For this review, use the dimensioned drawing (mm, ordinates from the lowest corner) and the shaded views. Give positions to 0.01 mm unless a question says otherwise; leave off trailing zeros. Write each loop counter-clockwise with the first axis right and the second up, starting at its lowest first coordinate (ties: lowest second). Pieces come first, ordered by that corner, then holes.
1) We need section D-D on x = 36. Give the boundary of the cut face in (y, z).
2) Draft analysis for pull direction Z (two halves, no side actions). For the marked faces 1 and 2, state which applies: pulls with the +Z half, pulls with the -Z half, needs draft (parallel to the pull), parting line crosses it, or undercut.
3) We need section B-B on x = 320. Give the boundary of the cut face in (y, z), and give its area (3 significant figures).
4) For P1, Ø11, axis at x = 307, z = 14.5, coming from the +Y side; P2, Ø6, axis at x = 317.5, y = 441.5, coming from the +Z side; P3, Ø11, axis at y = 101, z = 17, coming from the -X side; P4, Ø8, axis at x = 318, z = 14.5, coming from the -Y side, all flat-tipped, find the tip position at first contact; note any pin that passes through.
5) Wall thickness on line 1 along Y through (x, z) = (336, 12); line 2 along Z through (x, y) = (162, 141.5); line 3 along X through (y, z) = (475, 13.75): over which ranges is each line inside the solid? List them lowest first.
6) We need section C-C on y = 266. Give the boundary of the cut face in (x, z), and give its area (3 significant figures).
7) We need section A-A on z = 16.5. Give the boundary of the cut face in (x, y).
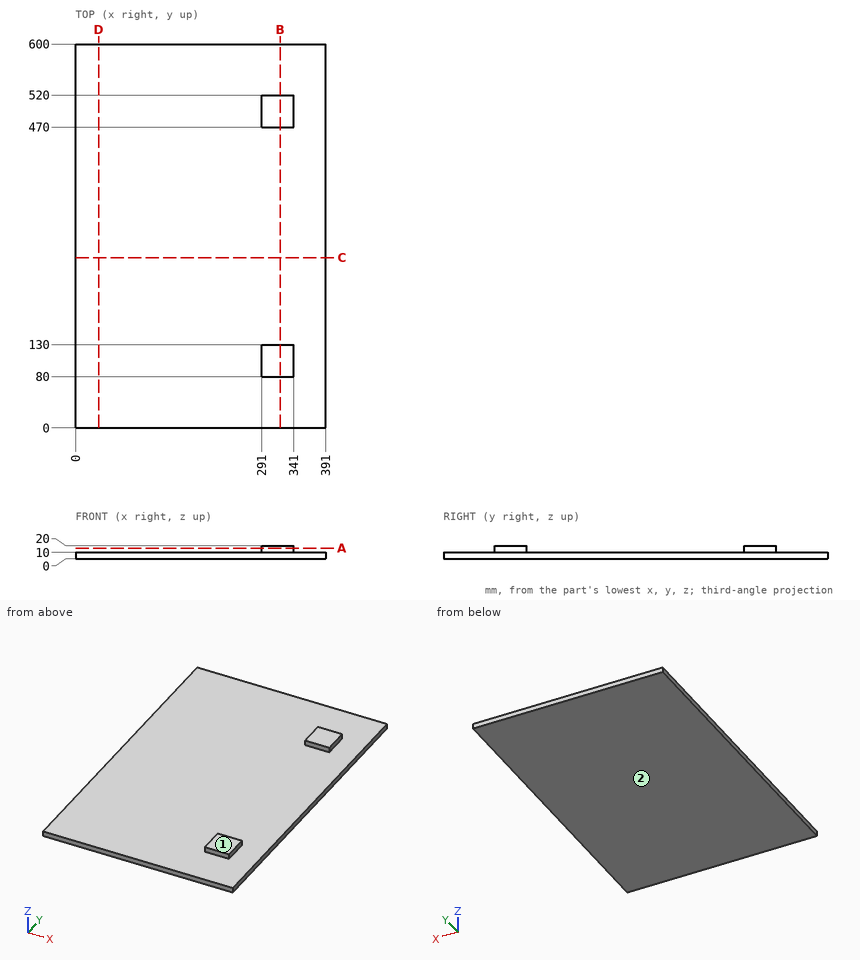
Results list:
1. outline: (0, 0) - (600, 0) - (600, 10) - (0, 10) - close
2. face 1: pulls with the +Z half
2. face 2: pulls with the -Z half
3. outline: (0, 0) - (600, 0) - (600, 10) - (520, 10) - (520, 20) - (470, 20) - (470, 10) - (130, 10) - (130, 20) - (80, 20) - (80, 10) - (0, 10) - close
3. area: 7,000 mm2
4. P1: stops at y = 600
4. P2: stops at z = 10
4. P3: stops at x = 291
4. P4: stops at y = 80
5. line 1: y = 80 to 130, 470 to 520
5. line 2: z = 0 to 10
5. line 3: x = 291 to 341
6. outline: (0, 0) - (391, 0) - (391, 10) - (0, 10) - close
6. area: 3,910 mm2
7. outline: (291, 80) - (341, 80) - (341, 130) - (291, 130) - close; (291, 470) - (341, 470) - (341, 520) - (291, 520) - close
